Read the model definition and answer for the solid it produces. Units are mm, in the model's axes. Coordinates: 2 decimals unless noted, no trailing zeros. Order: outer loops, then holes, each group sorted by start corner. A loop starts at its lowest first (then second) coordinate and runs counter-clockwise, first axis right, second up.
Autodesk Fusion 360 part; units mm, degrees
sketch "スケッチ1" plane through (0, 0, 0) normal (0, 1, 0) x (1, 0, 0)
  line L0 (57, 35) -> (-57, 35)
  line L1 (-57, 35) -> (-57, -35)
  line L2 (-57, -35) -> (57, -35)
  line L3 (57, -35) -> (57, 35)
  line L4 (57, 35) -> (-57, -35) construction
  line L5 (-57, 35) -> (57, -35) construction
  line L6 (61, 39) -> (-61, 39)
  line L7 (-61, 39) -> (-61, -39)
  line L8 (-61, -39) -> (61, -39)
  line L9 (61, -39) -> (61, 39)
  line L10 (61, 39) -> (-61, -39) construction
  line L11 (-61, 39) -> (61, -39) construction
  dimension "d9" = 114
  dimension "d10" = 70
  dimension "d11" = 78
  dimension "d12" = 122
extrude "押し出し1" add sketch "スケッチ1" along normal blind 4 contours L0 L1 L2 L3 | L6 L7 L8 L9
hole "穴1" at (-57, 0, -35) at (-57, 0, 35) at (57, 0, 35) at (57, 0, -35) direction (0, 1, 0) diameter 3.2 end through all
sketch "スケッチ2" plane through (0, 4, 0) normal (0, 1, 0) x (-1, 0, 0)
  circle A0 centre (-57, 35) radius 1.6
  circle A1 centre (57, -35) radius 1.6
  circle A2 centre (57, 35) radius 1.6
  circle A3 centre (-57, -35) radius 1.6
  line L0 (-61, 39) -> (-61, -39)
  line L1 (-61, -39) -> (61, -39)
  line L2 (61, -39) -> (61, 39)
  line L3 (61, 39) -> (-61, 39)
  line L4 (49, -19.5) -> (20, -19.5)
  line L5 (20, -19.5) -> (20, 29.5)
  line L6 (20, 29.5) -> (49, 29.5)
  line L7 (49, 29.5) -> (49, -19.5)
  line L8 (-12, -16) -> (-12, 26)
  line L9 (-44, -16) -> (-44, 26)
  point P0 (-12, 5)
  point P1 (-44, 5)
  point P2 (20, 5)
  dimension "d13" = 29
  dimension "d14" = 49
  dimension "d15" = 12
  dimension "d16" = 42
  dimension "d17" = 42
  dimension "d18" = 32
  dimension "d19" = 17
  dimension "d25" = 5
hole "穴2" at (-49, 4, -19.5) at (-49, 4, 29.5) at (-20, 4, 29.5) at (-20, 4, -19.5) at (44, 4, -16) at (44, 4, 26) at (12, 4, -16) at (12, 4, 26) direction (0, -1, 0) diameter 3 end through all
fillet "フィレット1" radius 1 4 edges at (61, 2, 39) (61, 2, -39) (-61, 2, 39) (-61, 2, -39)
1) A cutting plane is placed at B-B, the plane z = -16. Determine the outline of the cut face in (x, y).
A:
outline: (-61, 0) - (10.5, 0) - (10.5, 4) - (-61, 4) - close; (13.5, 0) - (42.5, 0) - (42.5, 4) - (13.5, 4) - close; (45.5, 0) - (61, 0) - (61, 4) - (45.5, 4) - close
2) A cutting plane is placed at A-A, the plane x = 44. Determine the outline of the cut face in (y, z), and give its area (3 significant figures).
A:
outline: (0, -39) - (4, -39) - (4, -17.5) - (0, -17.5) - close; (0, -14.5) - (4, -14.5) - (4, 24.5) - (0, 24.5) - close; (0, 27.5) - (4, 27.5) - (4, 39) - (0, 39) - close
area: 288 mm2
3) A flat-ended cylindrical pin translates along its axis: pin 1 Ø2.5 at (x, z) = (57, -35) entering from +Y. Find the tip coordinate at first contact, or state that the pin passes through.
A:
pin 1: passes through
4) Straight lines are drawn through the part: line 1 (X direction, y = 1.55, z = 29.5); line 2 (Z direction, x = -20, y = 3); line 3 (X direction, y = 2.75, z = 35). For each, find the intervals that lie inside material, in ascending order.
A:
line 1: x = -61 to -50.5, -47.5 to -21.5, -18.5 to 61
line 2: z = -39 to -21, -18 to 28, 31 to 39
line 3: x = -61 to -58.6, -55.4 to 55.4, 58.6 to 61
5) Determine the mould class of faces 1 (the flat face through (-61, 2, -1)), 2 (the cylindrical face through (56.93, 2.03, -33.4)), 3 (the flat face through (61, 2, 1)) for opening direction X: pulls with the +X half, pulls with the -X half, needs draft (parallel to the pull), parting line crosses it, or undercut.
A:
face 1: pulls with the -X half
face 2: undercut
face 3: pulls with the +X half
